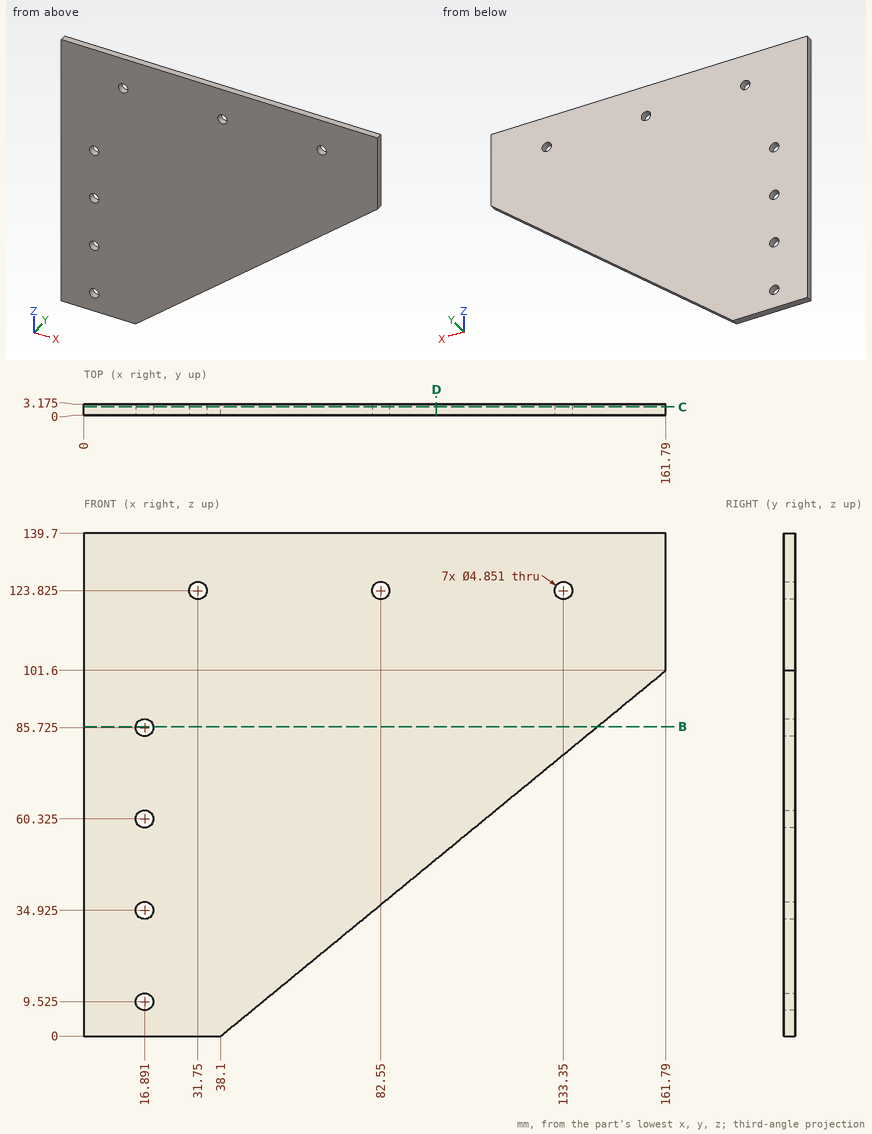
For this review, use the dimensioned drawing (mm, ordinates from the lowest corner) and the shaded views. Coordinates: 2 decimals unless noted, no trailing zeros. Order: outer loops, then holes, each group sorted by start corner. A loop starts at its lowest first (then second) coordinate and runs counter-clockwise, first axis right, second up. Notation, with made-up numbers: (27.25, -31.75) -> (47.25, -31.75) arc R33 cw to (47.25, -2.75) -> close; hole circle Ø8 at (-8, -25.75). An arc over 180 degrees is marked (long way). One line per item, written item: value. Start each with the question number.
Q1. Take a section at B-B, the plane z = 86. State the section outline as (x, y) points (1 decimal), then the cut area to 3 significant figures.
Q2. Insertion check: pin 1 Ø6.5 at (x, z) = (16.891, 85.725) entering from -Y; pin 2 Ø4.5 at (x, z) = (16.891, 9.525) entering from +Y; pin 3 Ø1 at (y, z) = (1, 92) entering from +X. Each pin has a flat end and moves straight along its axis. Give the tip position at first contact, or say it passes through.
Q3. Take a section at C-C, the plane y = 2.4. Give the number of separate pieces and of enclosed holes in the cut face, then the cut area to 3 significant figures.
Q4. Take a section at D-D, the plane x = 98. State the section outline as (y, z) points (1 decimal).
Q5. For probe 1 along Z at (x, y) = (17, 1.85); probe 2 along X at (y, z) = (1.05, 123); probe 3 along X at (y, z) = (0.15, 10) (1 decimal), list the stretches that pass through material, from the lowest coordinate up.
Values follow:
1. outline: (0, 0) -> (14.5, 0) -> (14.5, 3.2) -> (0, 3.2) -> close; (19.3, 0) -> (142.8, 0) -> (142.8, 3.2) -> (19.3, 3.2) -> close
1. area: 438 mm2
2. pin 1: stops at y = 0
2. pin 2: passes through
2. pin 3: stops at x = 150.71
3. separate pieces: 1
3. enclosed holes: 7
3. area: 16,200 mm2
4. outline: (0, 49.2) -> (3.2, 49.2) -> (3.2, 139.7) -> (0, 139.7) -> close
5. probe 1: z = 0 to 7.1, 11.95 to 32.5, 37.35 to 57.9, 62.75 to 83.3, 88.15 to 139.7
5. probe 2: x = 0 to 29.47, 34.03 to 80.27, 84.83 to 131.07, 135.63 to 161.79
5. probe 3: x = 0 to 14.5, 19.3 to 50.3
